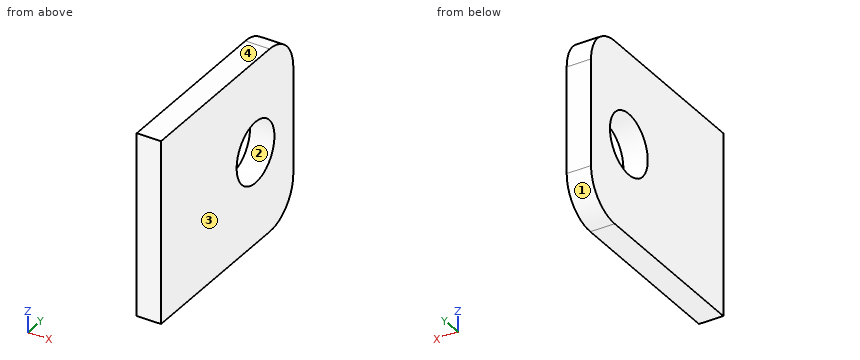
Autodesk Inventor part; units mm, degrees
ref_plane "YZ Plane" through (0, 0, 0) normal (1, 0, 0) x (0, 1, 0)
ref_plane "XZ Plane" through (0, 0, 0) normal (0, 1, 0) x (-1, 0, 0)
ref_plane "XY Plane" through (0, 0, 0) normal (0, 0, 1) x (1, 0, 0)
sketch "Sketch1" plane through (0, 0, 0) normal (1, 0, 0) x (0, 1, 0)
  circle A0 centre (0, 0) radius 2.54
  line L0 (5.08, 7.62) -> (-12.7, 7.62)
  line L1 (-12.7, 7.62) -> (-12.7, -7.62)
  line L2 (-12.7, -7.62) -> (5.08, -7.62)
  line L3 (5.08, -7.62) -> (5.08, 7.62)
  point P0 (5.08, 0)
  dimension "d0" = 5.08
  dimension "d1" = 15.24
  dimension "d2" = 17.78
  dimension "d5" = 5.08
extrude "Extrusion1" add sketch "Sketch1" along normal blind 2.032
fillet "Fillet1" radius 3.175 2 edges at (1.016, 5.08, 7.62) (1.016, 5.08, -7.62)
properties part number "Ell-Tab_small"
Verification items for the finished model (mm, model axes). Face numbers are marked on the shaded views. Coordinates: 2 decimals unless noted, no trailing zeros. Loops run counter-clockwise (first coordinate to the right, second up) from the corner with the lowest first, then second, coordinate; pieces in that order, holes last. Notation, with made-up numbers: (34.25, -33) -> (38.25, -33) arc R20 cw to (38.25, 5) -> close; hole circle Ø10 at (85.5, 7). An arc over 180 degrees is marked (long way). Write each question's results on one line, items separated by ' | '.
Item 1: Section check B-B, the plane z = 0. Enter the section's corners in (x, y), plus the area to 3 significant figures.
Found:
outline: (0, -12.7) -> (2.03, -12.7) -> (2.03, -2.54) -> (0, -2.54) -> close; (0, 2.54) -> (2.03, 2.54) -> (2.03, 5.08) -> (0, 5.08) -> close | area: 25.8 mm2
Item 2: Section check D-D, the plane z = -6.5. Enter the section's corners in (x, y), plus the area to 3 significant figures.
Found:
outline: (0, -12.7) -> (2.03, -12.7) -> (2.03, 4.33) -> (0, 4.33) -> close | area: 34.6 mm2
Item 3: Material ranges on L1, parallel to Z at x = 0.7, y = 0; L2, parallel to Y at x = 0.3, z = 1.25; L3, parallel to Y at x = 0.9, z = -0.5, recorded low to high.
Found:
L1: z = -7.62 to -2.54, 2.54 to 7.62 | L2: y = -12.7 to -2.21, 2.21 to 5.08 | L3: y = -12.7 to -2.49, 2.49 to 5.08
Item 4: Mould release check, pull along Z, two halves, no side actions. Record for the marked faces 1, 2, 3 and 4: +Z half, -Z half, draft (parallel to the pull), parting line (faces both ways), or undercut.
Found:
face 1: -Z half | face 2: undercut | face 3: draft | face 4: +Z half
Item 5: Section check C-C, the plane x = 1.2. Enter the section's corners in (y, z) (3 decimals).
Found:
outline: (-12.7, -7.62) -> (1.905, -7.62) arc R3.175 ccw to (5.08, -4.445) -> (5.08, 4.445) arc R3.175 ccw to (1.905, 7.62) -> (-12.7, 7.62) -> close; hole circle Ø5.08 at (0, 0)
Item 6: Section check A-A, the plane y = 0. Enter the section's corners in (x, z), plus the area to 3 significant figures.
Found:
outline: (0, -7.62) -> (2.03, -7.62) -> (2.03, -2.54) -> (0, -2.54) -> close; (0, 2.54) -> (2.03, 2.54) -> (2.03, 7.62) -> (0, 7.62) -> close | area: 20.6 mm2
